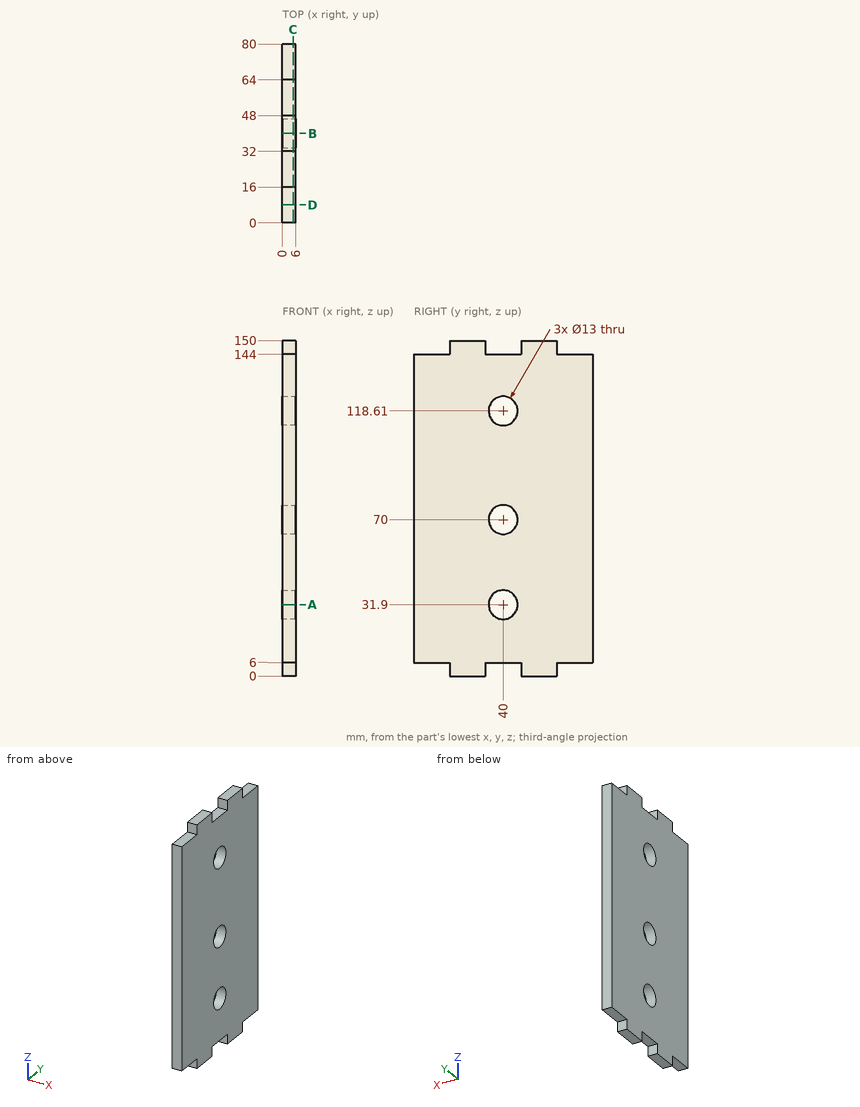
Here's the drawing with two shaded views (mm, measured from the low corner). I have some questions. Round coordinates to 2 decimals unless told otherwise and drop trailing zeros. Loops run counter-clockwise (first coordinate to the right, second up) from the corner with the lowest first, then second, coordinate; pieces in that order, holes last. Notation, with made-up numbers: (-32.5, -33) - (10.5, -33) arc R11 cw to (10.5, -21) - close; hole circle Ø2 at (-24, 37.5). An arc over 180 degrees is marked (long way). Use CSV: the item, a comma, the result in double quotes.
Item 1: If we section it at C-C on x = 4.8: List the corners of the cut face in (y, z) for me.
Here are the results:
outline,"(0, 6) - (16, 6) - (16, 0) - (32, 0) - (32, 6) - (48, 6) - (48, 0) - (64, 0) - (64, 6) - (80, 6) - (80, 144) - (64, 144) - (64, 150) - (48, 150) - (48, 144) - (32, 144) - (32, 150) - (16, 150) - (16, 144) - (0, 144) - close; hole circle Ø13 at (40, 31.9); hole circle Ø13 at (40, 70); hole circle Ø13 at (40, 118.61)"
Item 2: If we section it at A-A on z = 31.9: List the corners of the cut face in (x, y) for me.
Here are the results:
outline,"(0, 0) - (6, 0) - (6, 33.5) - (0, 33.5) - close; (0, 46.5) - (6, 46.5) - (6, 80) - (0, 80) - close"
Item 3: If we section it at B-B on y = 40: List the corners of the cut face in (x, z) for me, then the cut area to 3 significant figures.
Here are the results:
outline,"(0, 6) - (6, 6) - (6, 25.4) - (0, 25.4) - close; (0, 38.4) - (6, 38.4) - (6, 63.5) - (0, 63.5) - close; (0, 76.5) - (6, 76.5) - (6, 112.11) - (0, 112.11) - close; (0, 125.11) - (6, 125.11) - (6, 144) - (0, 144) - close"
area,"594 mm²"
Item 4: If we section it at D-D on y = 8: List the corners of the cut face in (x, z) for me.
Here are the results:
outline,"(0, 6) - (6, 6) - (6, 144) - (0, 144) - close"
Item 5: I need wall thicknesses on L1, parallel to Y at x = 1.3, z = 70; L2, parallel to Z at x = 1.75, y = 41.5; L3, parallel to Z at x = 3.3, y = 76.5. Which ranges of each line are inside material? Lowest first, please. Write a range as [from, to].
Here are the results:
L1,"y = [0, 33.5], [46.5, 80]"
L2,"z = [6, 25.58], [38.22, 63.68], [76.32, 112.29], [124.93, 144]"
L3,"z = [6, 144]"
Item 6: Will these pins go through, and if not, where does the flat tip stop? pin 1 (1.8 mm diameter, centred on x = 4, y = 68.5, fed in from +Z); pin 2 (3 mm diameter, centred on x = 3, y = 72, fed in from -Z); pin 3 (1.8 mm diameter, centred on x = 3, z = 2.5, fed in from -Y); pin 4 (8 mm diameter, centred on y = 40, z = 70, fed in from -X).
Here are the results:
pin 1,"stops at z = 144"
pin 2,"stops at z = 6"
pin 3,"stops at y = 16"
pin 4,"passes through"
